Part model, mm, in its own coordinate system. A direction names the side the tool comes from. Round coordinates to 2 decimals unless told otherwise and drop trailing zeros. Loops run counter-clockwise (first coordinate to the right, second up) from the corner with the lowest first, then second, coordinate; pieces in that order, holes last. Notation, with made-up numbers: (78, 81.5) -> (124, 81.5) arc R34 ccw to (124, 117.5) -> close; hole circle Ø9 at (-16, 80.5). An arc over 180 degrees is marked (long way). Answer as a JSON object with one key per item and string values. Group by question number.
from build123d import *

# Parameters (mm, degrees)
F0_R     = 20.047266
F1_DEPTH = 2.54


with BuildPart() as f1:
    # F0 (on Top) → F1 (new body)
    with BuildSketch(Plane.XY):
        with BuildLine():
            ThreePointArc((47.216884, 5.001183), (41.077621, 23.813338), (27.803349, 38.489217))
            Line((27.803349, 38.489217), (32.972034, 57.228676))
            Line((32.972034, 57.228676), (19.137083, 43.453631))
            ThreePointArc((19.137083, 43.453631), (-0.008949, 47.481006), (-19.153462, 43.446414))
            Line((-19.153462, 43.446414), (-32.759971, 56.977294))
            Line((-32.759971, 56.977294), (-27.926999, 38.399593))
            ThreePointArc((-27.926999, 38.399593), (-41.076878, 23.814619), (-47.200233, 5.155968))
            Line((-47.200233, 5.155968), (-66.047504, -0.059719))
            Line((-66.047504, -0.059719), (-47.209021, -5.074873))
            ThreePointArc((-47.209021, -5.074873), (-41.1448, -23.697077), (-28.080388, -38.287568))
            Line((-28.080388, -38.287568), (-32.963799, -56.859614))
            Line((-32.963799, -56.859614), (-19.379036, -43.346268))
            ThreePointArc((-19.379036, -43.346268), (-0.043958, -47.480986), (19.298742, -43.382076))
            Line((19.298742, -43.382076), (33.07547, -57.168957))
            Line((33.07547, -57.168957), (27.900469, -38.418873))
            ThreePointArc((27.900469, -38.418873), (41.109245, -23.758703), (47.217551, -4.994882))
            Line((47.217551, -4.994882), (65.72377, -0.11768))
            Line((65.72377, -0.11768), (47.216884, 5.001183))
        make_face()
        with BuildLine():
            Line((-43.119181, -6.163664), (-21.170047, -12.00693))
            Line((-21.170047, -12.00693), (-27.000214, -34.17957))
            ThreePointArc((-27.000214, -34.17957), (-37.754538, -21.722095), (-43.119181, -6.163664))
        make_face(mode=Mode.SUBTRACT)
        with BuildLine():
            Line((-16.37804, -40.36105), (0, -24.069112))
            Line((0, -24.069112), (16.308193, -40.389323))
            ThreePointArc((16.308193, -40.389323), (-0.037676, -43.557469), (-16.37804, -40.36105))
        make_face(mode=Mode.SUBTRACT)
        with BuildLine():
            Line((26.778455, -34.353586), (20.610804, -12.00693))
            Line((20.610804, -12.00693), (43.13225, -6.071539))
            ThreePointArc((43.13225, -6.071539), (37.707363, -21.803884), (26.778455, -34.353586))
        make_face(mode=Mode.SUBTRACT)
        Circle(F0_R, mode=Mode.SUBTRACT)
        with BuildLine():
            Line((-26.858221, 34.29126), (-21.153839, 12.3639))
            Line((-21.153839, 12.3639), (-43.100875, 6.290401))
            ThreePointArc((-43.100875, 6.290401), (-37.677324, 21.855749), (-26.858221, 34.29126))
        make_face(mode=Mode.SUBTRACT)
        with BuildLine():
            Line((43.123499, 6.133382), (20.597509, 12.3639))
            Line((20.597509, 12.3639), (26.683107, 34.427697))
            ThreePointArc((26.683107, 34.427697), (37.661421, 21.883142), (43.123499, 6.133382))
        make_face(mode=Mode.SUBTRACT)
        with BuildLine():
            Line((16.130895, 40.460459), (0, 24.399411))
            Line((0, 24.399411), (-16.145114, 40.454787))
            ThreePointArc((-16.145114, 40.454787), (-0.007654, 43.557485), (16.130895, 40.460459))
        make_face(mode=Mode.SUBTRACT)
    extrude(amount=F1_DEPTH)


solid = f1.part
Item 1: Band-saw the part on A-A, the plane x = 4. List the corners of the cut face in (y, z), plus the area to 3 significant figures.
Item 2: Which spindle directions (+Z, -Z, +X, -X, +Y, -Y) get a long thin tool onto all of the face, cutting with end or side? Do faces 4 (the face through (31.71, -9.08, 1.25)), 5 (the face through (-25.861, 50.117, 1.252)), 6 (the face through (30.524, -47.925, 1.252)), 7 (the face through (0, 21, 0)). Say none if no direction does.
Item 3: Band-saw the part on B-B, the plane y = 29. List the corners of the cut face in (x, z), plus the area to 3 significant figures.
Item 4: Band-saw the part on C-C, the plane x = 25. List the corners of the cut face in (y, z).
Item 5: Drill centre lines: line 1 (Y direction, x = 0, z = 0.8); line 2 (X direction, y = -34, z = 1.95); line 3 (X direction, y = -27.5, z = 0.2). Where is each one in solid material? Low to high.
Item 6: Band-saw the part on D-D, the plane y = -49. List the corners of the cut face in (x, z).
Item 7: Two-plate mould, pull along X, no slides. Class faces 1 (the face through (41.2, 23.6, 1.3)), 2 (the face through (-30.488, -47.444, 1.252)), 3 (the face through (-24.044, -22.938, 1.252)): pulls with the +X half, pulls with the -X half, needs draft (parallel to the pull), parting line crosses it, or undercut.
Entries:
{
 "1": {"outline": "(-47.31, 0) -> (-43.37, 0) -> (-43.37, 2.54) -> (-47.31, 2.54) -> close; (-28.07, 0) -> (-19.64, 0) -> (-19.64, 2.54) -> (-28.07, 2.54) -> close; (19.64, 0) -> (28.38, 0) -> (28.38, 2.54) -> (19.64, 2.54) -> close; (43.37, 0) -> (47.31, 0) -> (47.31, 2.54) -> (43.37, 2.54) -> close", "area": "63.6 mm²"},
 "2": {"face 4": "+Z, -Z", "face 5": "+Z, -Z, +Y", "face 6": "+Z, -Z, +X", "face 7": "-Z, +X, -X, +Y, -Y"},
 "3": {"outline": "(-37.6, 0) -> (-32.5, 0) -> (-32.5, 2.54) -> (-37.6, 2.54) -> close; (-25.48, 0) -> (-4.63, 0) -> (-4.63, 2.54) -> (-25.48, 2.54) -> close; (4.62, 0) -> (25.19, 0) -> (25.19, 2.54) -> (4.62, 2.54) -> close; (32.5, 0) -> (37.6, 0) -> (37.6, 2.54) -> (32.5, 2.54) -> close", "area": "131 mm²"},
 "4": {"outline": "(-49.09, 0) -> (-27.91, 0) -> (-27.91, 2.54) -> (-49.09, 2.54) -> close; (-10.85, 0) -> (11.15, 0) -> (11.15, 2.54) -> (-10.85, 2.54) -> close; (28.33, 0) -> (49.29, 0) -> (49.29, 2.54) -> (28.33, 2.54) -> close"},
 "5": {"line 1": "-47.48 to -43.56, -24.07 to -20.05, 20.05 to 24.4, 43.56 to 47.48", "line 2": "-33.14 to -27.23, -26.95 to -9.98, 9.92 to 26.68, 27.23 to 33.14", "line 3": "-38.71 to -33.78, -25.24 to -3.45, 3.43 to 24.89, 33.78 to 38.71"},
 "6": {"outline": "(-30.9, 0) -> (-25.06, 0) -> (-25.06, 2.54) -> (-30.9, 2.54) -> close; (24.91, 0) -> (30.82, 0) -> (30.82, 2.54) -> (24.91, 2.54) -> close"},
 "7": {"face 1": "pulls with the +X half", "face 2": "pulls with the -X half", "face 3": "undercut"}
}
